Study the drawing (mm; zero at the part's minimum x, y, z) and answer. A direction names the side the tool comes from. Round coordinates to 2 decimals unless told otherwise and drop trailing zeros. Order: outer loops, then holes, each group sorted by start corner. A loop starts at its lowest first (then second) coordinate and runs counter-clockwise, first axis right, second up. Notation, with made-up numbers: (-17.5, -8) - (34.5, -8) arc R21 cw to (34.5, 10) - close; hole circle Ø1 at (39.25, 21.5). An arc over 180 degrees is marked (long way). Use one line per item in the form item = value. Start each with the question number.
Q1. The part is cut by section A-A on x = 58.5. Determine the outline of the cut face in (y, z) (1 decimal), plus the area to 3 significant figures.
Q2. Which of the six approach directions +Z, -Z, +X, -X, +Y, -Y give full straight-line access (tool end or side, diameter ignored) to the marked faces 4 and 5?
Q3. For a pull along X with two mould halves and no side action, classify the marked faces 1, 2 and 3 as +X half, -X half, draft (parallel to the pull), parting line (faces both ways), or undercut.
Q4. The part is cut by section C-C on y = 84. Determine the outline of the cut face in (x, z) (1 decimal), plus the area to 3 significant figures.
Q5. Given P1, Ø10, axis at x = 89, z = 39, coming from the -Y side (1 decimal); P2, Ø2, axis at x = 25, z = 26.5, coming from the -Y side; P3, Ø4, axis at y = 62.5, z = 79.5, coming from the +X side; P4, Ø12, axis at x = 32, y = 44.5, coming from the +Z side, each flat-ended and moving along its own axis, determine where each tip first touches the part or whether it passes through.
Q6. The part is cut by section D-D on z = 15. Determine the outline of the cut face in (x, y).
Q7. The part is cut by section B-B on y = 48.5. Determine the outline of the cut face in (x, z) (1 decimal).
Q8. Find the intervals of material crossed by line 1 (Z direction, x = 19, y = 22); line 2 (Y direction, x = 46, z = 6.5) (1 decimal); line 3 (X direction, y = 55, z = 84) (1 decimal), in increasing order. Write a range as [from, to].
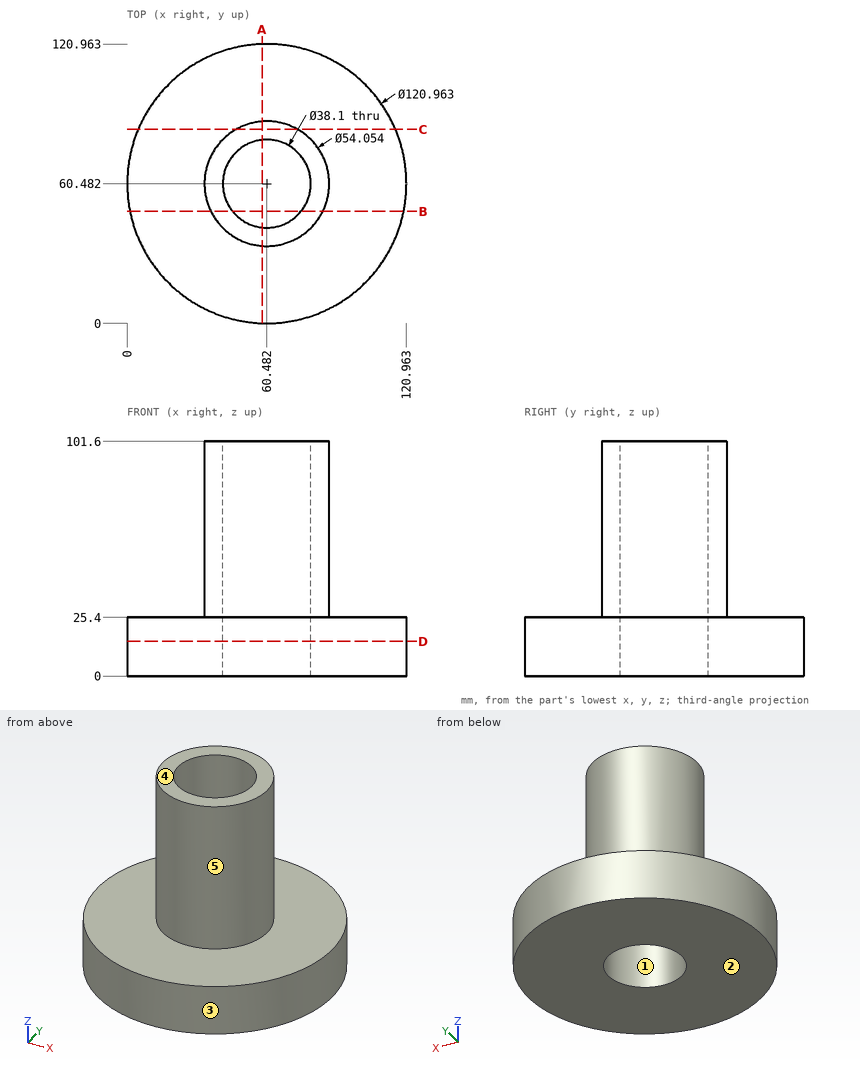
Found:
q1.outline = (0, 0) - (41.5, 0) - (41.5, 101.6) - (33.5, 101.6) - (33.5, 25.4) - (0, 25.4) - close; (79.4, 0) - (120.9, 0) - (120.9, 25.4) - (87.4, 25.4) - (87.4, 101.6) - (79.4, 101.6) - close
q1.area = 3,330 mm²
q2.face_4 = +Z, +X, -X, +Y, -Y
q2.face_5 = +Z
q3.face_1 = undercut
q3.face_2 = draft
q3.face_3 = parting line
q4.outline = (4.8, 0) - (116.2, 0) - (116.2, 25.4) - (73.8, 25.4) - (73.8, 101.6) - (47.2, 101.6) - (47.2, 25.4) - (4.8, 25.4) - close
q4.area = 4,860 mm²
q5.P1 = 47.2
q5.P2 = through
q5.P3 = 87.51
q5.P4 = 101.6
q6.outline = circle Ø120.96 at (60.48, 60.48); hole circle Ø38.1 at (60.48, 60.48)
q7.outline = (1.2, 0) - (45.7, 0) - (45.7, 101.6) - (36.3, 101.6) - (36.3, 25.4) - (1.2, 25.4) - close; (75.3, 0) - (119.8, 0) - (119.8, 25.4) - (84.7, 25.4) - (84.7, 101.6) - (75.3, 101.6) - close
q8.line_1 = [0, 25.4]
q8.line_2 = [1.8, 48.1], [72.9, 119.2]
q8.line_3 = [34, 42.2], [78.7, 86.9]
